Source: CAD feature listing. Evaluate the final solid. Frame: model axes, mm. A direction names the side the tool comes from. Give positions to 0.01 mm unless a question says otherwise; leave off trailing zeros. Loops run counter-clockwise (first coordinate to the right, second up) from the corner with the lowest first, then second, coordinate; pieces in that order, holes last.
from build123d import *

# Parameters (mm, degrees)
SKETCH1_W           = 74
SKETCH1_H           = 49
BOSS_EXTRUDE1_DEPTH = 7.9
FILLET1_R           = 5
CUT_EXTRUDE4_DEPTH  = 3.72
SKETCH3_R           = 1.65
CUT_EXTRUDE6_DEPTH  = 7.9
SKETCH7_W           = 22.1
SKETCH7_H           = 3.7
CUT_EXTRUDE7_DEPTH  = 3
SKETCH8_W           = 70.4
SKETCH8_H           = 45.4
CUT_EXTRUDE8_DEPTH  = 1.5
FILLET3_R           = 3
FILLET4_R           = 1
FILLET5_R           = 1
FILLET6_R           = 1


with BuildPart() as part:
    # Sketch1 → Boss-Extrude1 (new body)
    with BuildSketch(Plane(origin=(0, 0, 0), x_dir=(1, 0, 0), z_dir=(0, 1, 0))):
        Rectangle(SKETCH1_W, SKETCH1_H)
    extrude(amount=BOSS_EXTRUDE1_DEPTH)

    # Fillet1
    fillet1_edges = [part.edges().sort_by_distance(p)[0] for p in [
        (37, 3.95, 24.5),
        (-37, 3.95, 24.5),
        (-37, 3.95, -24.5),
        (37, 3.95, -24.5),
    ]]
    fillet(fillet1_edges, radius=FILLET1_R)

    # Sketch5 → Cut-Extrude4 (cut)
    with BuildSketch(Plane(origin=(0, 7.9, 0), x_dir=(1, 0, 0), z_dir=(0, 1, 0))):
        Polygon((-35.2, 15.9375), (-28.424, 15.9375), (-28.424, 21.171805633), (-28.424, 24.5), (28.424, 24.5), (28.424, 21.171805633), (28.424, 15.9375), (35.2, 15.9375), (35.2, -15.9375), (28.424, -15.9375), (28.424, -21.17), (-28.424, -21.17), (-28.424, -15.9375), (-35.2, -15.9375), align=None)
    extrude(amount=-CUT_EXTRUDE4_DEPTH, mode=Mode.SUBTRACT)

    # Sketch3 → Cut-Extrude6 (cut)
    with BuildSketch(Plane(origin=(0, 7.9, 0), x_dir=(1, 0, 0), z_dir=(0, 1, 0))):
        with Locations((-30.424, 17.9375)):
            Circle(SKETCH3_R)
        with Locations((30.424, 17.9375)):
            Circle(SKETCH3_R)
        with Locations((-30.424, -17.9375)):
            Circle(SKETCH3_R)
        with Locations((30.424, -17.9375)):
            Circle(SKETCH3_R)
    extrude(amount=-CUT_EXTRUDE6_DEPTH, mode=Mode.SUBTRACT)

    # Sketch7 → Cut-Extrude7 (cut)
    with BuildSketch(Plane.ZY.offset(37)):
        with Locations((0.7, 6.05)):
            Rectangle(SKETCH7_W, SKETCH7_H)
    extrude(amount=-CUT_EXTRUDE7_DEPTH, mode=Mode.SUBTRACT)

    # Sketch8 → Cut-Extrude8 (cut)
    with BuildSketch(Plane(origin=(0, 7.9, 0), x_dir=(1, 0, 0), z_dir=(0, 1, 0))):
        Rectangle(SKETCH8_W, SKETCH8_H)
    extrude(amount=-CUT_EXTRUDE8_DEPTH, mode=Mode.SUBTRACT)

    # Fillet3
    fillet3_edges = [part.edges().sort_by_distance(p)[0] for p in [
        (-35.2, 7.15, -22.7),
        (35.2, 7.15, -22.7),
        (-35.2, 7.15, 22.7),
        (35.2, 7.15, 22.7),
    ]]
    fillet(fillet3_edges, radius=FILLET3_R)

    # Fillet4
    fillet4_edges = [part.edges().sort_by_distance(p)[0] for p in [
        (-28.424, 5.29, -15.9375),
        (28.424, 5.29, -15.9375),
    ]]
    fillet(fillet4_edges, radius=FILLET4_R)

    # Fillet5
    fillet5_edges = [part.edges().sort_by_distance(p)[0] for p in [
        (28.424, 5.29, 15.9375),
        (-28.424, 5.29, 15.9375),
    ]]
    fillet(fillet5_edges, radius=FILLET5_R)

    # Fillet6
    fillet6_edges = [part.edges().sort_by_distance(p)[0] for p in [
        (-35.2, 6.05, -10.35),
        (-35.2, 6.05, 11.75),
    ]]
    fillet(fillet6_edges, radius=FILLET6_R)


solid = part.part
1) Contact query for flat-ended pins moving along their axis: P1, Ø3, axis at x = -30.42, z = 17.94, coming from the -Y side; P2, Ø1.9, axis at y = 6.5, z = 0, coming from the -X side; P3, Ø1.1, axis at x = 33.5, y = 5, coming from the -Z side; P4, Ø5.5, axis at x = 30.42, z = -17.94, coming from the +Y side. Output: stop coordinate, or through.
Checks:
P1: passes through
P2: stops at x = 35.2
P3: stops at z = -24.41
P4: stops at y = 6.4
2) Cut plane B-B (x = -24.5). Return loops of the section in (y, z).
Checks:
outline: (0, -24.5) - (4.18, -24.5) - (4.18, 21.17) - (6.4, 21.17) - (6.4, 22.7) - (7.9, 22.7) - (7.9, 24.5) - (0, 24.5) - close
3) Ray query, probe 1 along Z at (x, y) = (-31.5, 7.25); probe 2 along X at (y, z) = (6.75, -12.5); probe 3 along X at (y, z) = (1.75, 17). Return the intervals inside material, ascending.
Checks:
probe 1: z = -24.5 to -22.7, 22.7 to 24.5
probe 2: x = -37 to -35.2, 35.2 to 37
probe 3: x = -37 to -31.78, -29.07 to 29.07, 31.78 to 37
4) Reachability of faces 5 (the flat face through (0, 2, -24.5)), 6 (the cylindrical face through (34.34, 7.14, 21.8)) from +Z, -Z, +X, -X, +Y, -Y: full face, straight path, thin tool, end or side. Return the list, or none.
Checks:
face 5: -Z, +X, -X, +Y, -Y
face 6: +Y
5) Pull-direction query (Z, two-part tool) for faces 1 (the cylindrical face through (-35.57, 4.01, -23)), 2 (the cylindrical face through (-34.34, 7.14, -21.8)), 3 (the flat face through (28.424, 5, 19)), 4 (the flat face through (0, 4, 24.5)); classes: released by +Z, released by -Z, zero draft, split by the parting line, or undercut.
Checks:
face 1: released by -Z
face 2: undercut
face 3: zero draft
face 4: released by +Z
6) Cut plane C-C (y = 3.25). Return loops of the section in (x, z).
Checks:
outline: (-37, -19.5) arc R5 ccw to (-32, -24.5) - (32, -24.5) arc R5 ccw to (37, -19.5) - (37, 19.5) arc R5 ccw to (32, 24.5) - (-32, 24.5) arc R5 ccw to (-37, 19.5) - close; hole circle Ø3.3 at (-30.42, -17.94); hole circle Ø3.3 at (-30.42, 17.94); hole circle Ø3.3 at (30.42, -17.94); hole circle Ø3.3 at (30.42, 17.94)
